Verification items for the finished model (mm, model axes). Face numbers are marked on the shaded views. A direction names the side the tool comes from. Round coordinates to 2 decimals unless told otherwise and drop trailing zeros. Write each loop counter-clockwise with the first axis right and the second up, starting at its lowest first coordinate (ties: lowest second). Pieces come first, ordered by that corner, then holes. Notation, with made-up numbers: (50.25, -32.75) -> (81.25, -32.75) arc R19 cw to (81.25, -23.75) -> close; hole circle Ø7 at (-35, 35). An arc over 180 degrees is marked (long way). Use CSV: the item, a comma, the result in double quotes.
```python
from build123d import *

# Parameters (mm, degrees)
ESBO_O2_R                = 11
RESSALTO_EXTRUS_O1_DEPTH = 13
ESBO_O3_W                = 7
ESBO_O3_H                = 7
CORTE_EXTRUS_O1_DEPTH    = 26
CORTE_EXTRUS_O2_DEPTH    = 2.8
ESBO_O10_R               = 1.683661958
CORTE_EXTRUS_O3_DEPTH    = 2.8
ESBO_O11_R               = 11
ESBO_O11_R_2             = 9
RESSALTO_EXTRUS_O2_DEPTH = 2.5
CHANFRO1_SIZE            = 1


with BuildPart() as part:
    # Esboço2 → Ressalto-extrusão1 (new body)
    with BuildSketch(Plane(origin=(0, 0, 0), x_dir=(1, 0, 0), z_dir=(0, 1, 0))):
        with BuildLine():
            Line((-12.124355653, 7), (-37.124355653, 7))
            Line((-37.124355653, 7), (-37.124355653, -8.161034979))
            Line((-37.124355653, -8.161034979), (-11.375302548, -8.161034979))
            ThreePointArc((-11.375302548, -8.161034979), (13.982944229, 0.690847808), (-12.124355653, 7))
        make_face()
        Circle(ESBO_O2_R, mode=Mode.SUBTRACT)
    extrude(amount=RESSALTO_EXTRUS_O1_DEPTH)

    # Esboço3 → Corte-extrusão1 (cut)
    with BuildSketch(Plane.ZY.offset(37.124355653)):
        with Locations((0, 6.5)):
            Rectangle(ESBO_O3_W, ESBO_O3_H)
    extrude(amount=-CORTE_EXTRUS_O1_DEPTH, mode=Mode.SUBTRACT)

    # Esboço7 → Corte-extrusão2 (cut)
    with BuildSketch(Plane(origin=(0, 0, 3.5), x_dir=(-1, 0, 0), z_dir=(0, 0, -1))):
        Polygon((23.145814462, 6.5), (24.733527702, 3.75), (27.908954183, 3.75), (29.496667423, 6.5), (27.908954183, 9.25), (24.733527702, 9.25), align=None)
    extrude(amount=-CORTE_EXTRUS_O2_DEPTH, mode=Mode.SUBTRACT)

    # Esboço10 → Corte-extrusão3 (cut)
    with BuildSketch(Plane(origin=(0, 0, 6.3), x_dir=(-1, 0, 0), z_dir=(0, 0, -1))):
        with Locations((26.321240942, 6.5)):
            Circle(ESBO_O10_R)
    extrude(amount=-CORTE_EXTRUS_O3_DEPTH, mode=Mode.SUBTRACT)

    # Esboço11 → Ressalto-extrusão2 (add)
    with BuildSketch(Plane.XZ):
        Circle(ESBO_O11_R)
        Circle(ESBO_O11_R_2, mode=Mode.SUBTRACT)
    extrude(amount=-RESSALTO_EXTRUS_O2_DEPTH)

    # Chanfro1
    chanfro1_edges = [part.edges().sort_by_distance(p)[0] for p in [
        (-11, 13, 0),
    ]]
    chamfer(chanfro1_edges, length=CHANFRO1_SIZE)


solid = part.part
```
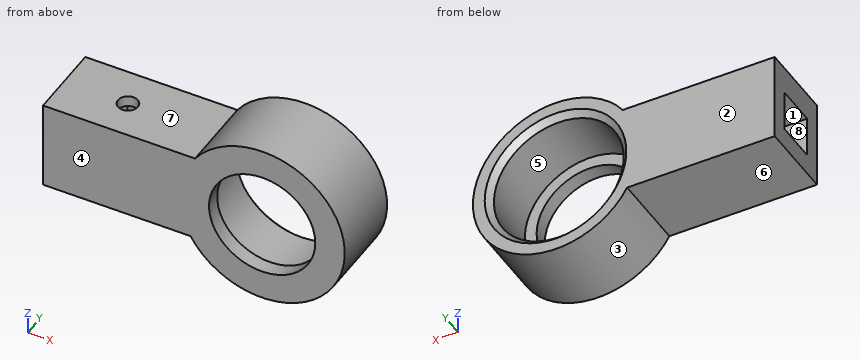
Q1. Mould release check, pull along Y, two halves, no side actions. Record for the marked faces 1, 2, 3 and 4: released by +Y, released by -Y, zero draft, split by the parting line, or undercut.
Filled in:
face 1,"undercut"
face 2,"released by +Y"
face 3,"zero draft"
face 4,"released by -Y"
Q2. Access from +Z, -Z, +X, -X, +Y, -Y to the whole of each face (thin tool, end or side, straight path). Record for the marked faces 5, 6, 7 and 8.
Filled in:
face 5,"+Y"
face 6,"-Z, -X, +Y, -Y"
face 7,"+Z, -X, +Y, -Y"
face 8,"-X"
Q3. Go/stop test with flat-tipped pins: P1, Ø3, axis at x = -27, y = 7.5, coming from the -Z side; P2, Ø2, axis at x = -26, y = 8, coming from the +Z side; P3, Ø4, axis at x = -3.5, y = 3.5, coming from the +Z side. Record where each tip stops, or that it passes through.
Filled in:
P1,"z = -7"
P2,"z = 8.16"
P3,"z = 13.92"
Q4. Section check D-D (y = 5.5). Record the cut outline in (x, z), plus the area to 3 significant figures.
Filled in:
outline,"(-37.12, -7) -> (-12.12, -7) arc R14 ccw (long way) to (-11.38, 8.16) -> (-24.97, 8.16) -> (-24.97, 6.3) -> (-23.72, 6.3) -> (-23.72, 3.5) -> (-11.12, 3.5) -> (-11.12, -3.5) -> (-37.12, -3.5) -> close; (-37.12, 3.5) -> (-28.92, 3.5) -> (-28.92, 6.3) -> (-27.68, 6.3) -> (-27.68, 8.16) -> (-37.12, 8.16) -> close; hole circle Ø22 at (0, 0)"
area,"396 mm²"
Q5. Section check B-B (x = 0). Record the cut outline in (y, z).
Filled in:
outline,"(0, -14) -> (13, -14) -> (13, -12) -> (12, -11) -> (2.5, -11) -> (2.5, -9) -> (0, -9) -> close; (0, 9) -> (2.5, 9) -> (2.5, 11) -> (12, 11) -> (13, 12) -> (13, 14) -> (0, 14) -> close"
Q6. Section check A-A (z = 0). Record the cut outline in (x, y).
Filled in:
outline,"(-37.12, 0) -> (-9, 0) -> (-9, 2.5) -> (-11, 2.5) -> (-11, 12) -> (-12, 13) -> (-37.12, 13) -> (-37.12, 10) -> (-11.12, 10) -> (-11.12, 3) -> (-37.12, 3) -> close; (9, 0) -> (14, 0) -> (14, 13) -> (12, 13) -> (11, 12) -> (11, 2.5) -> (9, 2.5) -> close"
Q7. Section check C-C (y = 1.5). Record the cut outline in (x, z).
Filled in:
outline,"(-37.12, -7) -> (-12.12, -7) arc R14 ccw (long way) to (-11.38, 8.16) -> (-37.12, 8.16) -> close; hole circle Ø18 at (0, 0)"
Q8. Material ranges on L1, parallel to Z at x = 0, y = 0.95; L2, parallel to Z at x = -22, y = 3.25; L3, parallel to X at y = 6.5, z = 5.5, recorded low to high.
Filled in:
L1,"-14 to -9, 9 to 14"
L2,"-7 to -3.5, 3.5 to 8.16"
L3,"-37.12 to -29.5, -23.15 to -9.53, 9.53 to 12.87"
